```python
from build123d import *

# Parameters (mm, degrees)
SKETCH_1_W          = 31
SKETCH_1_H          = 10
EXTRUDE_1_DEPTH     = 10
SKETCH_2_R          = 1.55
CUT_EXTRUDE_1_DEPTH = 20.111514854


with BuildPart() as part:
    # ｽｹｯﾁ1 → ﾎﾞｽ - 押し出し1 (new body)
    with BuildSketch(Plane(origin=(0, 0, 0), x_dir=(1, 0, 0), z_dir=(0, 1, 0))):
        Rectangle(SKETCH_1_W, SKETCH_1_H)
    extrude(amount=EXTRUDE_1_DEPTH)

    # ｽｹｯﾁ2 → ｶｯﾄ - 押し出し1 (cut, through all)
    with BuildSketch(Plane(origin=(0, 10, 0), x_dir=(1, 0, 0), z_dir=(0, 1, 0))):
        with Locations(Location((-10.5, 0, 0), (0, 0, 270))):
            Circle(SKETCH_2_R)
        with Locations(Location((10.5, 0, 0), (0, 0, 270))):
            Circle(SKETCH_2_R)
    extrude(amount=-CUT_EXTRUDE_1_DEPTH, mode=Mode.SUBTRACT)


solid = part.part
```
Work out the finished part from the listing and answer in its coordinate system (mm). Coordinates: 2 decimals unless noted, no trailing zeros. Write each loop counter-clockwise with the first axis right and the second up, starting at its lowest first coordinate (ties: lowest second). Pieces come first, ordered by that corner, then holes. Notation, with made-up numbers: (31.5, -37.75) - (44.5, -37.75) arc R21 cw to (44.5, -11.75) - close; hole circle Ø9 at (28.5, 66.25). An arc over 180 degrees is marked (long way). Answer as a JSON object with one key per item and string values.
Q1. For a pull along Z with two mould halves and no side action, classify faces 1 (the cylindrical face through (8.987, 5.07, -0.336)), 2 (the flat face through (15.5, 5, 0)), 3 (the flat face through (0, 5, 5)), 4 (the cylindrical face through (-12.013, 5.07, -0.336)) as pulls with the +Z half, pulls with the -Z half, needs draft (parallel to the pull), parting line crosses it, or undercut.
Results list:
{"face 1": "undercut", "face 2": "needs draft", "face 3": "pulls with the +Z half", "face 4": "undercut"}
Q2. Find section A-A (x = -10.5). Write down the section's boundary in (y, z), plus the area to 3 significant figures.
Results list:
{"outline": "(0, -5) - (10, -5) - (10, -1.55) - (0, -1.55) - close; (0, 1.55) - (10, 1.55) - (10, 5) - (0, 5) - close", "area": "69.0 mm^2"}
Q3. Find section C-C (y = 9). Write down the section's boundary in (x, z).
Results list:
{"outline": "(-15.5, -5) - (15.5, -5) - (15.5, 5) - (-15.5, 5) - close; hole circle Ø3.1 at (-10.5, 0); hole circle Ø3.1 at (10.5, 0)"}
Q4. Find section B-B (z = 0). Write down the section's boundary in (x, y).
Results list:
{"outline": "(-15.5, 0) - (-12.05, 0) - (-12.05, 10) - (-15.5, 10) - close; (-8.95, 0) - (8.95, 0) - (8.95, 10) - (-8.95, 10) - close; (12.05, 0) - (15.5, 0) - (15.5, 10) - (12.05, 10) - close"}
Q5. Given pin 1 Ø2.5 at (x, z) = (-10.5, 0) entering from -Y, flat-ended and moving along its own axis, determine where the tip first touches the part or whether it passes through.
Results list:
{"pin 1": "passes through"}
Q6. Consider L1, parallel to X at y = 4.75, z = 0; L2, parallel to Z at x = -11.5, y = 8.25. Determine where each line is inside the solid, lowest interval first. Write a range as from..to.
Results list:
{"L1": "x = -15.5..-12.05, -8.95..8.95, 12.05..15.5", "L2": "z = -5..-1.18, 1.18..5"}
